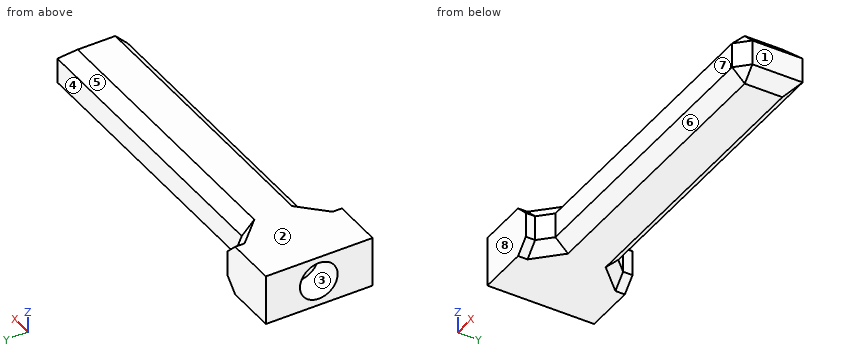
```python
from build123d import *

# Parameters (mm, degrees)
BASE_DEPTH         = 4
CHAMFER1_SIZE      = 1
SKETCH2_R          = 1.5
CUT_EXTRUDE1_DEPTH = 2.5


with BuildPart() as part:
    # Sketch1 → BASE (new body)
    with BuildSketch(Plane.XY):
        Polygon((0, -4.25), (0, -2.5), (25, -2.5), (25, 2.5), (0, 2.5), (0, 4.25), (-5, 4.25), (-5, -4.25), align=None)
    extrude(amount=BASE_DEPTH)

    # Chamfer1
    chamfer1_edges = [part.edges().sort_by_distance(p)[0] for p in [
        (0, -3.375, 0),
        (12.5, -2.5, 0),
        (25, 0, 0),
        (0, -3.375, 4),
        (0, 2.5, 2),
        (0, -2.5, 2),
        (25, -2.5, 2),
        (0, 3.375, 4),
        (12.5, 2.5, 4),
        (25, 0, 4),
        (12.5, 2.5, 0),
        (12.5, -2.5, 4),
        (0, 3.375, 0),
    ]]
    chamfer(chamfer1_edges, length=CHAMFER1_SIZE)

    # Sketch2 → Cut-Extrude1 (cut)
    with BuildSketch(Plane.ZY.offset(5)):
        with Locations((2.025680481, 0.035876769)):
            Circle(SKETCH2_R)
    extrude(amount=-CUT_EXTRUDE1_DEPTH, mode=Mode.SUBTRACT)


solid = part.part
```
The listing builds one solid part. Answer for the finished solid, in the listing's coordinates (mm). Face numbers are marked on the shaded views. A direction names the side the tool comes from. Round coordinates to 2 decimals unless told otherwise and drop trailing zeros. Loops run counter-clockwise (first coordinate to the right, second up) from the corner with the lowest first, then second, coordinate; pieces in that order, holes last. Notation, with made-up numbers: (42.25, 16) - (85.25, 16) arc R17 cw to (85.25, 37) - close; hole circle Ø8 at (22.25, -24.75). An arc over 180 degrees is marked (long way). Return JSON: item names as keys, results as strings. Group by question number.
1. Which of the six approach directions +Z, -Z, +X, -X, +Y, -Y give full straight-line access (tool end or side, diameter ignored) to the marked faces 4, 5, 6, 7 and 8?
2. The part is cut by section C-C on z = 1.9. Determine the outline of the cut face in (x, y).
3. The mould has two halves that part along Z. Classify the marked faces 1, 2 and 3: pulls with the +Z half, pulls with the -Z half, needs draft (parallel to the pull), parting line crosses it, or undercut.
4. Each of these flat-tipped pins is pushed along its axis until it touches: P1, Ø1.6, axis at x = 11.5, z = 2, coming from the +Y side; P2, Ø1.5, axis at y = 0.5, z = 1.5, coming from the -X side; P3, Ø0.6, axis at x = 12.5, z = 2.5, coming from the -Y side. Where does it stop, or does it pass through?
5. The part is cut by section A-A on x = 23. Determine the outline of the cut face in (y, z), then the cut area to 3 significant figures.
6. The part is cut by section B-B on y = 2. Determine the outline of the cut face in (x, z), then the cut area to 3 significant figures.
7. The part is cut by section D-D on y = -1. Determine the outline of the cut face in (x, z).
8. Consider probe 1 along Y at (x, z) = (12.5, 2.3); probe 2 along X at (y, z) = (-1, 1.6); probe 3 along Z at (x, y) = (-3.25, 1). Determine where each line is inside the solid, lowest interval first.
Resolved:
{
 "1": {"face 4": "+Z, -Z, +X, +Y", "face 5": "+Z, +X, +Y", "face 6": "-Z, +X, -Y", "face 7": "+Z, -Z, +X, -Y", "face 8": "+Z, -Z, +X, -X, -Y"},
 "2": {"outline": "(-5, -4.25) - (0, -4.25) - (0, -3.5) - (1, -2.5) - (24, -2.5) - (25, -1.5) - (25, 2.5) - (1, 2.5) - (0, 3.5) - (0, 4.25) - (-5, 4.25) - (-5, 1.53) - (-2.5, 1.53) - (-2.5, -1.46) - (-5, -1.46) - close"},
 "3": {"face 1": "needs draft", "face 2": "pulls with the +Z half", "face 3": "undercut"},
 "4": {"P1": "stops at y = 2.5", "P2": "stops at x = -2.5", "P3": "stops at y = -2.5"},
 "5": {"outline": "(-2.5, 1) - (-1.5, 0) - (1.5, 0) - (2.5, 1) - (2.5, 3) - (1.5, 4) - (-1.5, 4) - (-2.5, 3) - close", "area": "18.0 mm²"},
 "6": {"outline": "(-5, 0) - (0.5, 0) - (1, 0.5) - (24.5, 0.5) - (25, 1) - (25, 3) - (24.5, 3.5) - (1, 3.5) - (0.5, 4) - (-5, 4) - close", "area": "95.5 mm²"},
 "7": {"outline": "(-5, 0) - (24, 0) - (25, 1) - (25, 3) - (24, 4) - (-5, 4) - (-5, 3.11) - (-2.5, 3.11) - (-2.5, 0.94) - (-5, 0.94) - close"},
 "8": {"probe 1": "y = -2.5 to 2.5", "probe 2": "x = -2.5 to 25", "probe 3": "z = 0 to 0.88, 3.17 to 4"}
}
